Source: three-view drawing plus pictorial views. Frame: mm from the lowest corner of the part. Give positions to 0.01 mm unless a question says otherwise; leave off trailing zeros. Loops run counter-clockwise (first coordinate to the right, second up) from the corner with the lowest first, then second, coordinate; pieces in that order, holes last.
1. Material intervals for line 1 along Y through (x, z) = (92, 3.25); line 2 along X through (y, z) = (61, 2.95) (1 decimal); line 3 along Z through (x, y) = (32, 105.5), sorted ascending.
2. Section A-A, the plane y = 110. Output: boundary loops of the cut face in (x, z) (1 decimal).
3. Section C-C, the plane z = 3. Output: boundary loops of the cut face in (x, y) (1 decimal).
4. First-contact query: P1, Ø4, axis at x = 91.5, y = 34.5, coming from the +Z side. Flat tip, straight axial feed; report the tip coordinate or a pass-through.
5. Draft query along Y for the marked faces 1 and 2. Return one class per face: +Y half, -Y half, draft (parallel to the pull), parting line (faces both ways), or undercut.
6. Section B-B, the plane x = 40. Output: boundary loops of the cut face in (y, z), then the cut area to 3 significant figures.
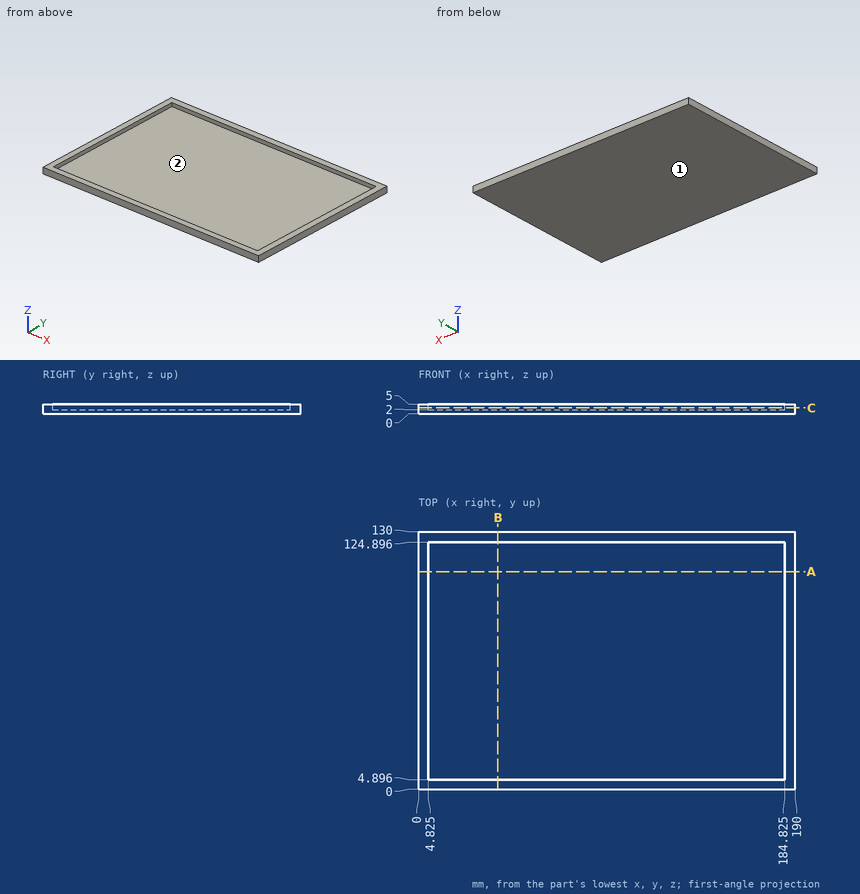
Answers below:
1. line 1: y = 0 to 4.9, 124.9 to 130
1. line 2: x = 0 to 4.8, 184.8 to 190
1. line 3: z = 0 to 2
2. outline: (0, 0) - (190, 0) - (190, 5) - (184.8, 5) - (184.8, 2) - (4.8, 2) - (4.8, 5) - (0, 5) - close
3. outline: (0, 0) - (190, 0) - (190, 130) - (0, 130) - close; hole (4.8, 4.9) - (184.8, 4.9) - (184.8, 124.9) - (4.8, 124.9) - close
4. P1: stops at z = 2
5. face 1: draft
5. face 2: undercut
6. outline: (0, 0) - (130, 0) - (130, 5) - (124.9, 5) - (124.9, 2) - (4.9, 2) - (4.9, 5) - (0, 5) - close
6. area: 290 mm2
